Could you check a few things on this model? Use its own coordinates, in mm. A direction names the side the tool comes from. Round coordinates to 2 decimals unless told otherwise and drop trailing zeros. One line per item, written item: value. Start each with the question number.
(1) I'm going to push a flat-ended pin straight in: pin 1 Ø22 at (x, y) = (457, 743) entering from -Z. Where does the tip first touch, or does it pass through?
(2) Thinking about a two-plate mould opening in X: for faces 3 (the face through (469, 773, 6)), 4 (the face through (379.58, 744.62, 14.01)), 5 (the face through (469.58, 744.62, 14.01)), which applies, released by +X, released by -X, zero draft, split by the parting line, or undercut?
(3) I want a section at A-A on y = 749.5. Count the separate pieces of the cut face and the enclosed holes in it, and give its area (3 significant figures).
(4) If I drill on L1, parallel to X at y = 749.5, z = 14.2; L2, parallel to X at y = 749.5, z = 13.8; L3, parallel to Y at x = 466.5, z = 11.5, over which ranges is the centre line in solid material (lowest first)?
(5) Which directions (+Z, -Z, +X, -X, +Y, -Y) give clear straight access to the entire face, cutting with the end or side of a thin tool? Please do faces 1 (the face through (469, 755, 13)), 2 (the face through (469, 755, 15)).
Autodesk Inventor part; units mm, degrees
ref_plane "Work Plane1" through (0, 0, 0) normal (0, 0, 1) x (1, 0, 0)
ref_plane "YZ Plane" through (0, 0, 0) normal (1, 0, 0) x (0, 1, 0)
ref_plane "XZ Plane" through (0, 0, 0) normal (0, 1, 0) x (-1, 0, 0)
ref_plane "Work Plane1" through (0, 0, 0) normal (0, 0, 1) x (1, 0, 0)
sketch "Sketch1" plane through (0, 0, 0) normal (0, 0, 1) x (1, 0, 0)
  line L0 (350.6597, 725) -> (590.6597, 725)
  line L1 (590.6597, 725) -> (590.6597, 775)
  line L2 (590.6597, 775) -> (350.6597, 775)
  line L3 (350.6597, 775) -> (350.6597, 725)
  line L4 (164.0316, 10) -> (164.0316, 1490)
  line L5 (777.2877, 10) -> (164.0316, 10)
  line L6 (470.6597, 10) -> (470.6597, 1506) construction
  line L7 (164.0316, 750) -> (680, 750) construction
  point P0 (0, 0)
  point P1 (470.6597, 725)
  point P2 (350.6597, 750)
  dimension "d0" = 240
  dimension "d1" = 50
extrude "Extrusion1" add sketch "Sketch1" along normal blind 15
sketch "Sketch2" plane through (350.6597, 725, 0) normal (-1, 0, 0) x (0, 0, 1)
  line L0 (15, 0) -> (0, 0)
  line L1 (0, 0) -> (0, 50)
  line L2 (0, 50) -> (15, 50)
  line L3 (15, 50) -> (15, 0)
  line L4 (12, 48) -> (0, 48)
  line L5 (0, 2) -> (12, 2)
  line L6 (13, 3) -> (13, 47)
  arc A0 (13, 47) -> (12, 48) centre (12, 47) ccw
  arc A1 (12, 2) -> (13, 3) centre (12, 3) ccw
  point P0 (0, -725)
  dimension "d5" = 2
extrude "Extrusion2" cut sketch "Sketch2" against normal through all contours L1 L4 A0 L6 A1 L5
fillet "Fillet1" radius 2 4 edges at (470.6597, 775, 15) (470.6597, 775, 0) (470.6597, 725, 0) (470.6597, 725, 15)
sketch "Sketch3" plane through (0, 0, 15) normal (0, 0, 1) x (1, 0, 0)
  line L0 (350.6597, 727) -> (590.6597, 727) construction
  line L1 (590.6597, 773) -> (590.6597, 727) construction
  line L2 (590.6597, 773) -> (350.6597, 773) construction
  line L3 (350.6597, 727) -> (350.6597, 773) construction
  line L4 (350.6597, 772) -> (590.6597, 772)
  line L5 (470.6597, 772) -> (470.6597, 727) construction
  circle A0 centre (470.6597, 749.5) radius 5
  point P0 (0, 0)
  dimension "d10" = 10
extrude "Extrusion3" cut sketch "Sketch3" against normal up to next
pattern_linear "Rectangular Pattern1" count 3 spacing 90 along (1, 0, 0) of "Extrusion3" first direction both ways yes
fillet "Fillet2" radius 2 14 edges at (350.6597, 725.5858, 14.4142) (350.6597, 725, 7.5) (350.6597, 725.5858, 0.5858) (350.6597, 774.4142, 14.4142) (350.6597, 775, 7.5) (350.6597, 774.4142, 0.5858) (350.6597, 750, 15) (590.6597, 774.4142, 14.4142) (590.6597, 775, 7.5) (590.6597, 774.4142, 0.5858) (590.6597, 725.5858, 14.4142) (590.6597, 725, 7.5) (590.6597, 725.5858, 0.5858) (590.6597, 750, 15)
properties part number "support3" material "Stainless Steel"
Found:
1. pin 1: stops at z = 13
2. face 3: zero draft
2. face 4: undercut
2. face 5: undercut
3. separate pieces: 4
3. enclosed holes: 0
3. area: 418 mm²
4. L1: x = 351.06 to 375.66, 385.66 to 465.66, 475.66 to 555.66, 565.66 to 590.26
4. L2: x = 350.83 to 375.66, 385.66 to 465.66, 475.66 to 555.66, 565.66 to 590.49
4. L3: y = 725 to 727, 773 to 775
5. face 1: -Z, +X, -X
5. face 2: +Z, +X, -X, +Y, -Y
